from build123d import *

# Parameters (mm, degrees)
F0_W            = 12.7
F0_H            = 12.7
F2_W            = 6
F2_H            = 25.4
F4_W            = 3.175
F4_H            = 7.2644
F5_DEPTH        = 63.501
F7_DEPTH        = 1.27
F7_COPIES_COUNT = 16


# Not quite as in the source:
# - a pattern or mirror of a feature is missing from the dataset's text; its kind, count and spacing are read off the source's solid


with BuildPart() as f1:
    # F0 (on Front) → F1 (revolve)
    with BuildSketch(Plane.XZ):
        Polygon((-50.8, 0), (0, 0), (0, 50.8), (-12.7, 50.8), (-31.75, 50.8), align=None)
        with Locations((-6.35, 57.15)):
            Rectangle(F0_W, F0_H)
    revolve(axis=Axis((0, 0, 25.4), (0, 0, 1)))

    # F2 (on Front) → F3 (revolve, cut)
    with BuildSketch(Plane.XZ):
        Polygon((-8.255, 38.1), (-38.1, 0), (0, 0), (0, 38.1), (-6, 38.1), align=None)
        with Locations((-3, 50.8)):
            Rectangle(F2_W, F2_H)
    revolve(axis=Axis((0, 0, 19.05), (0, 0, -1)), mode=Mode.SUBTRACT)

    # F4 (on Top) → F5 (cut, through all)
    with BuildSketch(Plane.XY):
        with Locations((0, 3.6322)):
            Rectangle(F4_W, F4_H)
    extrude(amount=F5_DEPTH, mode=Mode.SUBTRACT)

    # F6 (on Front) → F7 (cut, symmetric)
    with BuildSketch(Plane.XZ):
        Polygon((-12.7, 38.1), (-41.275, 0), (-34.925, 0), (-6.35, 38.1), align=None)
    f7 = extrude(amount=F7_DEPTH, both=True, mode=Mode.SUBTRACT)

    # F7_copies: F7 ×16 about axis
    f7_copies_axis = Axis((0, 0, 0), (0, 0, 1))
    for i in range(1, F7_COPIES_COUNT):
        add(f7.rotate(f7_copies_axis, i * 360 / F7_COPIES_COUNT), mode=Mode.SUBTRACT)


solid = f1.part
Geometry check sheet. Reference: the model listing, model coordinates, mm. Give positions to 0.01 mm unless a question says otherwise; leave off trailing zeros. Loops run counter-clockwise (first coordinate to the right, second up) from the corner with the lowest first, then second, coordinate; pieces in that order, holes last. Notation, with made-up numbers: M 50.25,84.25 L 62.25,84.25 A17 ccw 62.25,110.25 Z; hole C 10.25,88.25 d5. An arc over 180 degrees is marked long. Write each question's results on one line, items separated by ' | '.
1) Section check C-C, the plane y = 0. Record the boundary of the cut face in (x, z) (3 decimals), plus the area to 3 significant figures.
Answers follow:
outline: M -50.8,0 L -41.275,0 L -12.7,38.1 L -6,38.1 L -6,63.5 L -12.7,63.5 L -12.7,50.8 L -31.75,50.8 Z; M 6,38.1 L 12.7,38.1 L 41.275,0 L 50.8,0 L 31.75,50.8 L 12.7,50.8 L 12.7,63.5 L 6,63.5 Z | area: 2,150 mm2
2) Gauge pin test, flat ends, axial feed: pin 1 (4 mm diameter, centred on x = -14.5, z = 48.5, fed in from +Y); pin 2 (5 mm diameter, centred on x = 38, z = 20.5, fed in from -Y); pin 3 (15.5 mm diameter, centred on x = 0, y = 0, fed in from -Z). Record the tip position at first contact, or that the pin passes through.
Answers follow:
pin 1: y = 30.45 | pin 2: y = -24.82 | pin 3: z = 38.1
3) Section check A-A, the plane x = 0. Record the boundary of the cut face in (y, z) (3 decimals), plus the area to 3 significant figures.
Answers follow:
outline: M -50.8,0 L -41.275,0 L -12.7,38.1 L -6,38.1 L -6,63.5 L -12.7,63.5 L -12.7,50.8 L -31.75,50.8 Z; M 7.264,38.1 L 12.7,38.1 L 41.275,0 L 50.8,0 L 31.75,50.8 L 12.7,50.8 L 12.7,63.5 L 7.264,63.5 Z | area: 2,120 mm2
4) Release check for a two-part mould opening along Y. For faces 1 (the face through (2.75, 12.4, 57.24)), 2 (the face through (22.24, -14.78, 14.55)), 3 (the face through (-22.24, 14.78, 14.55)) record: +Y half, -Y half, draft (parallel to the pull), parting line (faces both ways), or undercut.
Answers follow:
face 1: parting line | face 2: undercut | face 3: undercut
5) Section check B-B, the plane z = 54.5. Record the boundary of the cut face in (x, y).
Answers follow:
outline: C 0,0 d25.4; hole M -1.59,5.79 A6 ccw long 1.59,5.79 L 1.59,7.26 L -1.59,7.26 Z
6) Thickness scan on line 1 (Y direction, x = 0, z = 53.5); line 2 (X direction, y = 0, z = 51); line 3 (Y direction, x = -11, z = 18). Record the ranges inside material, lowest first.
Answers follow:
line 1: -12.7 to -6, 7.26 to 12.7 | line 2: -12.7 to -6, 6 to 12.7 | line 3: -42.65 to -25.51, -23.24 to -21.33, 21.33 to 23.24, 25.51 to 42.65
